Read the model definition and answer for the solid it produces. Units are mm, in the model's axes. Face numbers are marked on the shaded views. A direction names the side the tool comes from. Coordinates: 2 decimals unless noted, no trailing zeros. Write each loop counter-clockwise with the first axis right and the second up, starting at its lowest first coordinate (ties: lowest second). Pieces come first, ordered by that corner, then holes. Notation, with made-up numbers: (19, -10) -> (33, -10) arc R21 cw to (33, 2) -> close; hole circle Ø11 at (74, 17). An arc over 180 degrees is marked (long way). Answer in a Markdown table with one row per item. Add a question column.
Item 1: Section D-D on x = 12.5 is taken. Write down the section's boundary in (y, z) (3 decimals), then the cut area to 3 significant figures.
Item 2: Section C-C on z = 30 is taken. Write down the section's boundary in (x, y), then the cut area to 3 significant figures.
Item 3: Straight lines are drawn through the part: line 1 (Y direction, x = 18.5, z = 12); line 2 (Y direction, x = 16, z = 14); line 3 (X direction, y = -16.5, z = 19). For each, find the intervals that lie inside material, in ascending order. Write a range as from..to.
Item 4: Section A-A on x = 17.5 is taken. Count the separate pieces of the cut face and the enclosed holes in it, then the cut area to 4 significant figures.
Item 5: Section B-B on y = -40 is taken. Write down the section's boundary in (x, z).
Item 6: For a pull along Y with two mould halves and no side action, classify the marked faces 3, 4 and 5 as +Y half, -Y half, draft (parallel to the pull), parting line (faces both ways), or undercut.
Item 7: Which of the six approach directions +Z, -Z, +X, -X, +Y, -Y give full straight-line access (tool end or side, diameter ignored) to the marked faces 1 and 2?
Item 8: Given pin 1 Ø6 at (x, z) = (17.5, 20) entering from +Y; pin 2 Ø3.5 at (x, z) = (17.5, 20) entering from -Y; pin 3 Ø3 at (x, y) = (9.5, 7) entering from +Z, each flat-ended and moving along its own axis, determine where each tip first touches the part or whether it passes through.
```python
from build123d import *

# Parameters (mm, degrees)
SKETCH1_W           = 35
SKETCH1_H           = 35
SKETCH1_W_2         = 26
SKETCH1_H_2         = 26
SKETCH1_H_3         = 30
SKETCH1_W_3         = 25
SKETCH1_H_4         = 15
BOSS_EXTRUDE2_DEPTH = 40
FILLET3_R           = 3.5
FILLET4_R           = 4
SKETCH6_R           = 2.3
CUT_EXTRUDE5_DEPTH  = 5
BOSS_EXTRUDE3_DEPTH = 40
SKETCH7_R           = 8
CUT_EXTRUDE8_DEPTH  = 10
SKETCH11_R          = 6.25
CUT_EXTRUDE9_DEPTH  = 4
SKETCH12_R          = 2.75
CUT_EXTRUDE10_DEPTH = 97.046863561
FILLET5_R           = 4


with BuildPart() as part:
    # Sketch1 → Boss-Extrude2 (new body)
    # profile 1 of 2: a face of its own
    with BuildSketch(Plane.XY):
        with Locations((17.5, 17.5)):
            Rectangle(SKETCH1_W, SKETCH1_H)
        with Locations((17.5, 17)):
            Rectangle(SKETCH1_W_2, SKETCH1_H_2, mode=Mode.SUBTRACT)
    # profile 2 of 2: a face of its own
    with BuildSketch(Plane.XY):
        with Locations((17.5, -15)):
            Rectangle(SKETCH1_W, SKETCH1_H_3)
        with Locations((17.5, -12.5)):
            Rectangle(SKETCH1_W_3, SKETCH1_H_4, mode=Mode.SUBTRACT)
    extrude(amount=BOSS_EXTRUDE2_DEPTH)

    # Fillet3
    fillet3_edges = [part.edges().sort_by_distance(p)[0] for p in [
        (4.5, 30, 20),
        (4.5, 4, 20),
        (30.5, 4, 20),
        (30.5, 30, 20),
    ]]
    fillet(fillet3_edges, radius=FILLET3_R)

    # Fillet4
    fillet4_edges = [part.edges().sort_by_distance(p)[0] for p in [
        (0, 35, 20),
        (35, 35, 20),
    ]]
    fillet(fillet4_edges, radius=FILLET4_R)

    # Sketch6 → Cut-Extrude5 (cut)
    with BuildSketch(Plane(origin=(0, 35, 0), x_dir=(1, 0, 0), z_dir=(0, 1, 0))):
        with Locations(Location((17.5, -20, 0), (0, 0, 270))):
            Circle(SKETCH6_R)
    extrude(amount=-CUT_EXTRUDE5_DEPTH, mode=Mode.SUBTRACT)

    # Sketch9 → Boss-Extrude3 (add)
    with BuildSketch(Plane.XY.offset(40)):
        Polygon((5, -30), (0, -30), (0, -52), (35, -52), (35, -30), (30, -30), (30, -45), (5, -45), align=None)
    extrude(amount=-BOSS_EXTRUDE3_DEPTH)

    # Sketch7 → Cut-Extrude8 (cut)
    with BuildSketch(Plane(origin=(0, -20, 0), x_dir=(1, 0, 0), z_dir=(0, 1, 0))):
        with Locations(Location((17.5, -20, 0), (0, 0, 180))):
            Circle(SKETCH7_R)
    extrude(amount=-CUT_EXTRUDE8_DEPTH, mode=Mode.SUBTRACT)

    # Sketch11 → Cut-Extrude9 (cut)
    with BuildSketch(Plane(origin=(0, -45, 0), x_dir=(1, 0, 0), z_dir=(0, 1, 0))):
        with Locations(Location((17.5, -20, 0), (0, 0, 270))):
            Circle(SKETCH11_R)
    extrude(amount=-CUT_EXTRUDE9_DEPTH, mode=Mode.SUBTRACT)

    # Sketch12 → Cut-Extrude10 (cut, through all)
    with BuildSketch(Plane(origin=(0, -45, 0), x_dir=(1, 0, 0), z_dir=(0, 1, 0))):
        with Locations(Location((17.5, -20, 0), (0, 0, 270))):
            Circle(SKETCH12_R)
    extrude(amount=-CUT_EXTRUDE10_DEPTH, mode=Mode.SUBTRACT)

    # Fillet5
    fillet5_edges = [part.edges().sort_by_distance(p)[0] for p in [
        (30, -5, 20),
        (5, -5, 20),
        (30, -30, 20),
        (5, -30, 20),
    ]]
    fillet(fillet5_edges, radius=FILLET5_R)


solid = part.part
```
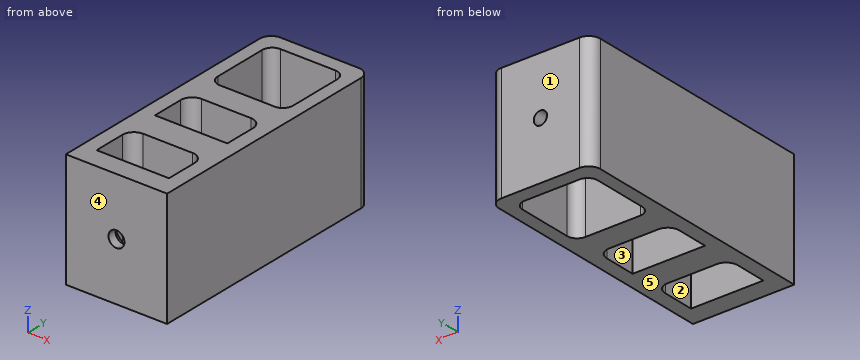
Results below:
| question | item | result |
|---|---|---|
| 1 | outline | (-52, 0) -> (-45, 0) -> (-45, 16.25) -> (-49, 16.25) -> (-49, 23.75) -> (-45, 23.75) -> (-45, 40) -> (-52, 40) -> close; (-30, 0) -> (-20, 0) -> (-20, 13.755) -> (-30, 13.755) -> close; (-30, 26.245) -> (-20, 26.245) -> (-20, 40) -> (-30, 40) -> close; (-5, 0) -> (4, 0) -> (4, 40) -> (-5, 40) -> close; (30, 0) -> (35, 0) -> (35, 40) -> (30, 40) -> close |
| 1 | area | 1,090 mm2 |
| 2 | outline | (0, -52) -> (35, -52) -> (35, 31) arc R4 ccw to (31, 35) -> (4, 35) arc R4 ccw to (0, 31) -> close; hole (4.5, 7.5) arc R3.5 ccw to (8, 4) -> (27, 4) arc R3.5 ccw to (30.5, 7.5) -> (30.5, 26.5) arc R3.5 ccw to (27, 30) -> (8, 30) arc R3.5 ccw to (4.5, 26.5) -> close; hole (5, -45) -> (30, -45) -> (30, -34) arc R4 ccw to (26, -30) -> (9, -30) arc R4 ccw to (5, -34) -> close; hole (5, -20) -> (30, -20) -> (30, -9) arc R4 ccw to (26, -5) -> (9, -5) arc R4 ccw to (5, -9) -> close |
| 2 | area | 1,640 mm2 |
| 3 | line 1 | y = -52..-45, -30..-20, -5..4, 30..35 |
| 3 | line 2 | y = -52..-49, -5..4, 30..35 |
| 3 | line 3 | x = 0..5, 30..35 |
| 4 | separate pieces | 7 |
| 4 | enclosed holes | 0 |
| 4 | area | 990.5 mm2 |
| 5 | outline | (0, 0) -> (5, 0) -> (5, 40) -> (0, 40) -> close; (30, 0) -> (35, 0) -> (35, 40) -> (30, 40) -> close |
| 6 | face 3 | undercut |
| 6 | face 4 | -Y half |
| 6 | face 5 | draft |
| 7 | face 1 | +Z, -Z, +X, -X, +Y |
| 7 | face 2 | +Z, -Z |
| 8 | pin 1 | stops at y = 35 |
| 8 | pin 2 | stops at y = -5 |
| 8 | pin 3 | passes through |
